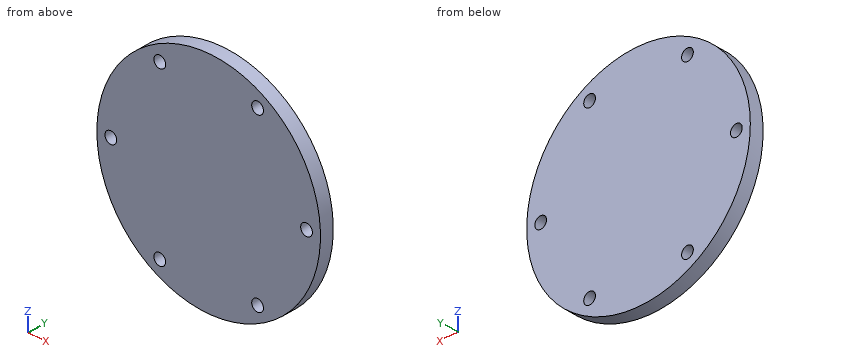
Autodesk Inventor part; units mm, degrees
ref_plane "YZ Plane" through (0, 0, 0) normal (1, 0, 0) x (0, 1, 0)
ref_plane "XZ Plane" through (0, 0, 0) normal (0, 1, 0) x (-1, 0, 0)
ref_plane "XY Plane" through (0, 0, 0) normal (0, 0, 1) x (1, 0, 0)
sketch "Sketch4" plane through (0, 0, 0) normal (0, 1, 0) x (-1, 0, 0)
  circle A0 centre (0, 0) radius 50.8
  dimension "d2" = 101.6
extrude "Extrusion3" add sketch "Sketch4" along normal blind 6.35
sketch "Sketch10" plane through (0, 6.35, 0) normal (0, 1, 0) x (1, 0, 0)
  circle A0 centre (-44.462, 0) radius 2.667
  circle A1 centre (-22.231, -38.5052) radius 2.667
  circle A2 centre (22.231, -38.5052) radius 2.667
  circle A3 centre (44.462, 0) radius 2.667
  circle A4 centre (22.231, 38.5052) radius 2.667
  circle A5 centre (-22.231, 38.5052) radius 2.667
  point P0 (0, 0)
  dimension "d48" = 5.334
  dimension "d51" = 360
extrude "Extrusion6" cut sketch "Sketch10" against normal blind 6.35
properties part number "cap"
Here's how the part is built. I have some questions about the finished solid (model axes, mm). Coordinates: 2 decimals unless noted, no trailing zeros. Order: outer loops, then holes, each group sorted by start corner. A loop starts at its lowest first (then second) coordinate and runs counter-clockwise, first axis right, second up.
Item 1: I need wall thicknesses on probe 1 along Z at (x, y) = (24, 1); probe 2 along X at (y, z) = (1.25, -37); probe 3 along X at (y, z) = (1.75, 38). Which ranges of each line are inside material? Lowest first, please.
Response values:
probe 1: z = -44.77 to -40.5, -36.51 to 36.51, 40.5 to 44.77
probe 2: x = -34.81 to -24.43, -20.03 to 20.03, 24.43 to 34.81
probe 3: x = -33.71 to -24.85, -19.61 to 19.61, 24.85 to 33.71
Item 2: If we section it at A-A, the plane z = 0: List the corners of the cut face in (x, y) for me (3 decimals), then the cut area to 3 significant figures.
Response values:
outline: (-50.8, 0) - (-47.129, 0) - (-47.129, 6.35) - (-50.8, 6.35) - close; (-41.795, 0) - (41.795, 0) - (41.795, 6.35) - (-41.795, 6.35) - close; (47.129, 0) - (50.8, 0) - (50.8, 6.35) - (47.129, 6.35) - close
area: 577 mm2
Item 3: I'm going to push flat-ended pins straight in: pin 1 Ø3 at (x, y) = (26, 1.5) entering from -Z; pin 2 Ø1.5 at (y, z) = (1, 34) entering from +X; pin 3 Ø1.5 at (x, y) = (-9, 4) entering from +Z; pin 4 Ø5 at (x, z) = (-22.23, 38.51) entering from +Y. Where does each tip first touch, or does it pass through?
Response values:
pin 1: stops at z = -44.5
pin 2: stops at x = 38.41
pin 3: stops at z = 50.13
pin 4: passes through
Item 4: If we section it at B-B, the plane y = 4.5: List the corners of the cut face in (x, z) for me (3 decimals).
Response values:
outline: circle Ø101.6 at (0, 0); hole circle Ø5.334 at (-44.462, 0); hole circle Ø5.334 at (-22.231, -38.505); hole circle Ø5.334 at (-22.231, 38.505); hole circle Ø5.334 at (22.231, -38.505); hole circle Ø5.334 at (22.231, 38.505); hole circle Ø5.334 at (44.462, 0)
Item 5: If we section it at D-D, the plane z = -28.5: List the corners of the cut face in (x, y) for me.
Response values:
outline: (-42.05, 0) - (42.05, 0) - (42.05, 6.35) - (-42.05, 6.35) - close
Item 6: If we section it at C-C, the plane x = -15: List the corners of the cut face in (y, z) for me, then the cut area to 3 significant figures.
Response values:
outline: (0, -48.53) - (6.35, -48.53) - (6.35, 48.53) - (0, 48.53) - close
area: 616 mm2
